Can you work these out from the model? Positions are in its coordinate system, mm. A direction names the side the tool comes from. Round coordinates to 2 decimals unless told otherwise and drop trailing zeros. Loops run counter-clockwise (first coordinate to the right, second up) from the corner with the lowest first, then second, coordinate; pieces in that order, holes last. Notation, with made-up numbers: (25, -30.75) -> (55, -30.75) arc R25 cw to (55, -10.75) -> close; hole circle Ø11 at (27.25, 70). An arc over 180 degrees is marked (long way). Answer as a JSON object with one key per item and string values.
Autodesk Inventor part; units mm, degrees
ref_plane "YZ Plane" through (0, 0, 0) normal (1, 0, 0) x (0, 1, 0)
ref_plane "XZ Plane" through (0, 0, 0) normal (0, 1, 0) x (-1, 0, 0)
ref_plane "XY Plane" through (0, 0, 0) normal (0, 0, 1) x (1, 0, 0)
sketch "Sketch1" plane through (0, 0, 0) normal (0, 0, 1) x (1, 0, 0)
  line L0 (-84.0204, 0) -> (84.0204, 0)
  line L1 (0, -84.0204) -> (0, 84.0204)
  arc A0 (-4, 11.8427) -> (4, 11.8427) centre (0, 0) ccw
  line L2 (0, 16) -> (4, 16)
  line L3 (4, 16) -> (4, 11.8427)
  line L4 (0, 16) -> (-4, 16)
  line L5 (-4, 16) -> (-4, 11.8427)
  circle A1 centre (0, 0) radius 25
  circle A2 centre (0, 0) radius 38 construction
  arc A3 (18.541, 57.0634) -> (16.0059, 57.8257) centre (0, 0) ccw
  circle A4 centre (32.909, 19) radius 5
  line L6 (32.909, 19) -> (0, 0) construction
  circle A5 centre (-32.909, 19) radius 5
  circle A6 centre (0, -38) radius 5
  line L7 (0, 60) -> (0, 52)
  line L8 (0, 52) -> (16.0059, 57.8257)
  line L9 (18.541, 57.0634) -> (16.0689, 49.4549)
  line L10 (-16.0689, 49.4549) -> (-2.6466, 59.9416)
  arc A7 (0, 60) -> (-2.6466, 59.9416) centre (0, 0) ccw
  line L11 (0, 60) -> (0, 52)
  line L12 (-30.5648, 42.0689) -> (-21.04, 56.19)
  arc A8 (-18.541, 57.0634) -> (-21.04, 56.19) centre (0, 0) ccw
  line L13 (-18.541, 57.0634) -> (-16.0689, 49.4549)
  line L14 (-42.0689, 30.5648) -> (-37.3739, 46.9382)
  arc A9 (-35.2671, 48.541) -> (-37.3739, 46.9382) centre (0, 0) ccw
  line L15 (-35.2671, 48.541) -> (-30.5648, 42.0689)
  line L16 (-49.4549, 16.0689) -> (-50.0494, 33.0917)
  arc A10 (-48.541, 35.2671) -> (-50.0494, 33.0917) centre (0, 0) ccw
  line L17 (-48.541, 35.2671) -> (-42.0689, 30.5648)
  line L18 (-52, 0) -> (-57.8257, 16.0059)
  arc A11 (-57.0634, 18.541) -> (-57.8257, 16.0059) centre (0, 0) ccw
  line L19 (-57.0634, 18.541) -> (-49.4549, 16.0689)
  line L20 (-49.4549, -16.0689) -> (-59.9416, -2.6466)
  arc A12 (-60, 0) -> (-59.9416, -2.6466) centre (0, 0) ccw
  line L21 (-60, 0) -> (-52, 0)
  line L22 (-42.0689, -30.5648) -> (-56.19, -21.04)
  arc A13 (-57.0634, -18.541) -> (-56.19, -21.04) centre (0, 0) ccw
  line L23 (-57.0634, -18.541) -> (-49.4549, -16.0689)
  line L24 (-30.5648, -42.0689) -> (-46.9382, -37.3739)
  arc A14 (-48.541, -35.2671) -> (-46.9382, -37.3739) centre (0, 0) ccw
  line L25 (-48.541, -35.2671) -> (-42.0689, -30.5648)
  line L26 (-16.0689, -49.4549) -> (-33.0917, -50.0494)
  arc A15 (-35.2671, -48.541) -> (-33.0917, -50.0494) centre (0, 0) ccw
  line L27 (-35.2671, -48.541) -> (-30.5648, -42.0689)
  line L28 (0, -52) -> (-16.0059, -57.8257)
  arc A16 (-18.541, -57.0634) -> (-16.0059, -57.8257) centre (0, 0) ccw
  line L29 (-18.541, -57.0634) -> (-16.0689, -49.4549)
  line L30 (16.0689, -49.4549) -> (2.6466, -59.9416)
  arc A17 (0, -60) -> (2.6466, -59.9416) centre (0, 0) ccw
  line L31 (0, -60) -> (0, -52)
  line L32 (30.5648, -42.0689) -> (21.04, -56.19)
  arc A18 (18.541, -57.0634) -> (21.04, -56.19) centre (0, 0) ccw
  line L33 (18.541, -57.0634) -> (16.0689, -49.4549)
  line L34 (42.0689, -30.5648) -> (37.3739, -46.9382)
  arc A19 (35.2671, -48.541) -> (37.3739, -46.9382) centre (0, 0) ccw
  line L35 (35.2671, -48.541) -> (30.5648, -42.0689)
  line L36 (49.4549, -16.0689) -> (50.0494, -33.0917)
  arc A20 (48.541, -35.2671) -> (50.0494, -33.0917) centre (0, 0) ccw
  line L37 (48.541, -35.2671) -> (42.0689, -30.5648)
  line L38 (52, 0) -> (57.8257, -16.0059)
  arc A21 (57.0634, -18.541) -> (57.8257, -16.0059) centre (0, 0) ccw
  line L39 (57.0634, -18.541) -> (49.4549, -16.0689)
  line L40 (49.4549, 16.0689) -> (59.9416, 2.6466)
  arc A22 (60, 0) -> (59.9416, 2.6466) centre (0, 0) ccw
  line L41 (60, 0) -> (52, 0)
  line L42 (42.0689, 30.5648) -> (56.19, 21.04)
  arc A23 (57.0634, 18.541) -> (56.19, 21.04) centre (0, 0) ccw
  line L43 (57.0634, 18.541) -> (49.4549, 16.0689)
  line L44 (30.5648, 42.0689) -> (46.9382, 37.3739)
  arc A24 (48.541, 35.2671) -> (46.9382, 37.3739) centre (0, 0) ccw
  line L45 (48.541, 35.2671) -> (42.0689, 30.5648)
  line L46 (16.0689, 49.4549) -> (33.0917, 50.0494)
  arc A25 (35.2671, 48.541) -> (33.0917, 50.0494) centre (0, 0) ccw
  line L47 (35.2671, 48.541) -> (30.5648, 42.0689)
  point P0 (0, -12.5)
  point P1 (-2, 16)
  point P2 (17.305, 53.2592)
  point P3 (0, 56)
  point P4 (-17.305, 53.2592)
  point P5 (-32.916, 45.305)
  point P6 (-45.305, 32.916)
  point P7 (-53.2592, 17.305)
  point P8 (-56, 0)
  point P9 (-53.2592, -17.305)
  point P10 (-45.305, -32.916)
  point P11 (-32.916, -45.305)
  point P12 (-17.305, -53.2592)
  point P13 (0, -56)
  point P14 (17.305, -53.2592)
  point P15 (32.916, -45.305)
  point P16 (45.305, -32.916)
  point P17 (53.2592, -17.305)
  point P18 (56, 0)
  point P19 (53.2592, 17.305)
  point P20 (45.305, 32.916)
  point P21 (32.916, 45.305)
  point P22 (-60, 0)
  point P23 (0, -60)
  point P24 (60, 0)
  dimension "d4" = 76
  dimension "d0" = 25
  dimension "d1" = 8
  dimension "d2" = 28.5
  dimension "d3" = 50
  dimension "d5" = 120
  dimension "d6" = 10
  dimension "d7" = 60
  dimension "d10" = 360
  dimension "d12" = 8
  dimension "d13" = 70
  dimension "d14" = 8
  dimension "d15" = 18
  dimension "d19" = 360
  dimension "d21" = 17.0332
extrude "Extrusion1" add sketch "Sketch1" along normal mid plane 22 contours A1 L1 L4 L5 A0 L0 | L0 A0 L1 A1 | A1 L0 A0 L3 L2 L1 | L1 A0 L0 A1
extrude "Extrusion2" add sketch "Sketch1" along normal mid plane 10 contours L0 A1 L1 A6 L28 A16 L29 L26 A15 L27 L24 A14 L25 L22 A13 L23 L20 A12 | L18 A11 L19 L16 A10 L17 L14 A9 L15 L12 A8 L13 L10 A7 L1 A1 L0 | L1 L8 A3 L9 L46 A25 L47 L44 A24 L45 L42 A23 L43 L40 A22 L0 A1 | A1 L0 L38 A21 L39 L36 A20 L37 L34 A19 L35 L32 A18 L33 L30 A17 L1 A6
fillet "Fillet1" radius 2 2 edges at (-25, 0, 5) (-25, 0, -5)
chamfer "Chamfer1" distance 1.5 angle 45 2 edges at (0, -12.5, 11) (0, -12.5, -11) measured on face at (-4.9522, 11.4772, 3.6667)
properties part number "Piesa 35"
Q1. I'm going to push flat-ended pins straight in: pin 1 (9 mm diameter, centred on x = 54, z = 2, fed in from -Y); pin 2 (13 mm diameter, centred on x = 32.909, y = 19, fed in from -Z); pin 3 (3.5 mm diameter, centred on y = 13.5, z = 3, fed in from +X). Where does each tip first touch, or does it pass through?
Determined:
{"pin 1": "y = -33.91", "pin 2": "z = -5", "pin 3": "x = 52.83"}
Q2. If I drill on L1, parallel to Z at x = 26.5, y = -22.5; L2, parallel to X at y = -9.5, z = -8; L3, parallel to Y at x = -47, z = 3, over which ranges is the centre line in solid material (lowest first)? Write a range as [from, to].
Determined:
{"L1": "[-5, 5]", "L2": "[-23.12, -8.12], [8.12, 23.12]", "L3": "[-37.3, -34.15], [-27.24, 34.15]"}
Q3. I want a section at B-B, the plane y = 29. Write out the boundary of the cut face in (x, z), then the cut area to 3 significant figures.
Determined:
{"outline": "(-49.91, -5) -> (44.39, -5) -> (44.39, 5) -> (-49.91, 5) -> close", "area": "943 mm²"}
Q4. On a 3-axis mill with a long thin cutter (end or side, diameter ignored), from which of +Z, -Z, +X, -X, +Y, -Y can I reach the whole of each face in a straight line? I mean faces 5 (the flat face through (-49.03, -25.87, -0.07)), 6 (the flat face through (4, 14, 0)), 7 (the flat face through (53.31, 17.32, -0.07)), 8 (the cylindrical face through (23.846, -7.509, 8.972)), 9 (the flat face through (-45.35, 32.95, -0.07)). Say none if no direction works.
Determined:
{"face 5": "+Z, -Z, -X", "face 6": "+Z, -Z", "face 7": "+Z, -Z, +X", "face 8": "+Z", "face 9": "+Z, -Z, +Y"}
Q5. We'd pull the mould along X, two halves only. Please class faces 1 (the flat face through (-45.35, -32.95, -0.07)), 2 (the cylindrical face through (-0.651, -42.957, -0.07)), 3 (the flat face through (-56, 0, 0)), 4 (the flat face through (32.95, 45.35, -0.07)): pulls with the +X half, pulls with the -X half, needs draft (parallel to the pull), parting line crosses it, or undercut.
Determined:
{"face 1": "pulls with the -X half", "face 2": "undercut", "face 3": "needs draft", "face 4": "pulls with the +X half"}
Q6. I want a section at A-A, the plane z = -2.5. Give the number of separate pieces and of enclosed holes in the cut face, then the cut area to 3 significant figures.
Determined:
{"separate pieces": "1", "enclosed holes": "4", "area": "9,160 mm²"}
